Geometry check sheet. Reference: the model listing, model coordinates, mm. A direction names the side the tool comes from. Coordinates: 2 decimals unless noted, no trailing zeros. Write each loop counter-clockwise with the first axis right and the second up, starting at its lowest first coordinate (ties: lowest second). Pieces come first, ordered by that corner, then holes. Notation, with made-up numbers: (80.5, 78) -> (88.5, 78) arc R31 ccw to (88.5, 111) -> close; hole circle Ø4 at (6, 49). An arc over 180 degrees is marked (long way). Use a Markdown table: item, result.
Autodesk Inventor part; units mm, degrees
ref_plane "YZ Plane" through (0, 0, 0) normal (1, 0, 0) x (0, 1, 0)
ref_plane "XZ Plane" through (0, 0, 0) normal (0, 1, 0) x (-1, 0, 0)
ref_plane "XY Plane" through (0, 0, 0) normal (0, 0, 1) x (1, 0, 0)
sketch "Sketch1" plane through (0, 0, 0) normal (0, 0, 1) x (1, 0, 0)
  line L0 (-10, -110) -> (10, -110)
  line L1 (10, -110) -> (10, 110)
  line L2 (10, 110) -> (-10, 110)
  line L3 (-10, 110) -> (-10, -110)
  point P0 (0, 0)
  dimension "width" = 20
  dimension "d1" = 10
  dimension "d2" = 220
  dimension "d3" = 110
extrude "Extrusion1" add sketch "Sketch1" along normal blind 5
sketch "Sketch4" plane through (-10, -110, 0) normal (-1, 0, 0) x (0, 0, 1)
  line L0 (5, 0) -> (5, 220)
  line L1 (0, 0) -> (5, 0)
  line L2 (5, 0) -> (5, 19.7)
  line L3 (5, 19.7) -> (0, 19.7)
  line L4 (0, 19.7) -> (0, 0)
  point P0 (0, 110)
  dimension "d29" = 19.7
extrude "Extrusion4" add sketch "Sketch4" along normal blind 5
mirror "Mirror1" about plane through (0, 0, 0) normal (0, 1, 0) of "Extrusion4"
properties part number "EBF_001.1-side-plate_cup-holder"
Item 1: Tool access check on faces 5 (the flat face through (0, 2, 0)), 6 (the flat face through (-10, 1, 2)). Record the directions out of +Z, -Z, +X, -X, +Y, -Y that give a thin tool (end or side, any length) a straight path to the whole face; none if there is none.
Answer block:
| item | result |
|---|---|
| face 5 | -Z, +X, -X, +Y, -Y |
| face 6 | +Z, -Z, -X |
Item 2: Depth check by flat-ended pin: P1, Ø2.5, axis at y = -30.5, z = 3, coming from the -X side. Enter the tip coordinate at first touch or a pass-through.
Answer block:
| item | result |
|---|---|
| P1 | stops at x = -10 |
Item 3: Thickness scan on L1, parallel to Y at x = -13.5, z = 0.8; L2, parallel to X at y = 70, z = 4. Record the ranges inside material, lowest first. Write a range as [from, to].
Answer block:
| item | result |
|---|---|
| L1 | y = [-110, -90.3], [90.3, 110] |
| L2 | x = [-10, 10] |
Item 4: Section check A-A on z = 2.55. Record the boundary of the cut face in (x, y), then the cut area to 3 significant figures.
Answer block:
| item | result |
|---|---|
| outline | (-15, -110) -> (10, -110) -> (10, 110) -> (-15, 110) -> (-15, 90.3) -> (-10, 90.3) -> (-10, -90.3) -> (-15, -90.3) -> close |
| area | 4,600 mm^2 |
Item 5: Section check B-B on y = 88. Record the boundary of the cut face in (x, z), then the cut area to 3 significant figures.
Answer block:
| item | result |
|---|---|
| outline | (-10, 0) -> (10, 0) -> (10, 5) -> (-10, 5) -> close |
| area | 100 mm^2 |
Item 6: Mould release check, pull along Y, two halves, no side actions. Record for faces 1 (the flat face through (-3, -110, 2)), 2 (the flat face through (-12, -90.3, 3)), 3 (the flat face through (-12, 90.3, 2)), 4 (the flat face through (10, -2, 2)): +Y half, -Y half, draft (parallel to the pull), parting line (faces both ways), or undercut.
Answer block:
| item | result |
|---|---|
| face 1 | -Y half |
| face 2 | undercut |
| face 3 | undercut |
| face 4 | draft |
